Check sheet for the modelled part. Datum: model origin and axes. Units: mm. A direction names the side the tool comes from. Coordinates: 2 decimals unless noted, no trailing zeros. Order: outer loops, then holes, each group sorted by start corner. A loop starts at its lowest first (then second) coordinate and runs counter-clockwise, first axis right, second up.
from build123d import *

# Parameters (mm, degrees)
SKETCH1_R           = 5
SKETCH1_R_2         = 2.5
BOSS_EXTRUDE1_DEPTH = 12
SKETCH2_R           = 5
BOSS_EXTRUDE2_DEPTH = 1
FILLET1_R           = 1


with BuildPart() as part:
    # Sketch1 → Boss-Extrude1 (new body)
    with BuildSketch(Plane(origin=(0, 0, 0), x_dir=(0, 0, -1), z_dir=(1, 0, 0))):
        Circle(SKETCH1_R)
        Circle(SKETCH1_R_2, mode=Mode.SUBTRACT)
    extrude(amount=BOSS_EXTRUDE1_DEPTH)

    # Sketch2 → Boss-Extrude2 (add)
    with BuildSketch(Plane(origin=(12, 0, 0), x_dir=(0, 0, -1), z_dir=(1, 0, 0))):
        Circle(SKETCH2_R)
    extrude(amount=BOSS_EXTRUDE2_DEPTH)

    # Fillet1
    fillet1_edges = [part.edges().sort_by_distance(p)[0] for p in [
        (13, 0, 5),
    ]]
    fillet(fillet1_edges, radius=FILLET1_R)


solid = part.part
(1) Cross-section at C-C (x = 8). Enter the section's corners in (y, z).
Filled in:
outline: circle Ø10 at (0, 0); hole circle Ø5 at (0, 0)
(2) Thickness scan on probe 1 along Y at (x, z) = (4.75, 0); probe 2 along X at (y, z) = (2.25, 1); probe 3 along Z at (x, y) = (10, -3). Record the ranges inside material, lowest first.
Filled in:
probe 1: y = -5 to -2.5, 2.5 to 5
probe 2: x = 12 to 13
probe 3: z = -4 to 4
(3) Cross-section at A-A (y = 0). Enter the section's corners in (x, z).
Filled in:
outline: (0, -5) - (12, -5) arc R1 ccw to (13, -4) - (13, 4) arc R1 ccw to (12, 5) - (0, 5) - (0, 2.5) - (12, 2.5) - (12, -2.5) - (0, -2.5) - close
(4) Tool access check on faces 1 (the flat face through (12, 0, 0)), 2 (the cylindrical face through (5.92, -4.88, 1.08)). Record the directions out of +Z, -Z, +X, -X, +Y, -Y that give a thin tool (end or side, any length) a straight path to the whole face; none if there is none.
Filled in:
face 1: -X
face 2: +X, -X
(5) Go/stop test with flat-tipped pins: P1, Ø4, axis at x = 10, z = -2.5, coming from the +Y side; P2, Ø3, axis at x = 10, y = 2, coming from the +Z side. Record where each tip stops, or that it passes through.
Filled in:
P1: stops at y = 4.97
P2: stops at z = 4.97
